from build123d import *

# Parameters (mm, degrees)
SKETCH1_W           = 700
SKETCH1_H           = 20
BOSS_EXTRUDE1_DEPTH = 2
FILLET1_R           = 9
SKETCH2_R           = 5
SKETCH2_R_2         = 2.25
CUT_EXTRUDE1_DEPTH  = 701.288511972


with BuildPart() as part:
    # Sketch1 → Boss-Extrude1 (new body)
    with BuildSketch(Plane(origin=(0, 0, 0), x_dir=(1, 0, 0), z_dir=(0, 1, 0))):
        with Locations((350, 10)):
            Rectangle(SKETCH1_W, SKETCH1_H)
    extrude(amount=BOSS_EXTRUDE1_DEPTH)

    # Fillet1
    fillet1_edges = [part.edges().sort_by_distance(p)[0] for p in [
        (0, 1, -20),
        (700, 1, -20),
        (700, 1, 0),
        (0, 1, 0),
    ]]
    fillet(fillet1_edges, radius=FILLET1_R)

    # Sketch2 → Cut-Extrude1 (cut, through all)
    with BuildSketch(Plane(origin=(0, 2, 0), x_dir=(1, 0, 0), z_dir=(0, 1, 0))):
        with Locations(Location((350, 10, 0), (0, 0, 270))):
            Circle(SKETCH2_R)
        with Locations(Location((130, 15, 0), (0, 0, 270))):
            Circle(SKETCH2_R_2)
        with Locations(Location((230, 15, 0), (0, 0, 270))):
            Circle(SKETCH2_R_2)
        with Locations(Location((130, 5, 0), (0, 0, 270))):
            Circle(SKETCH2_R_2)
        with Locations(Location((230, 5, 0), (0, 0, 270))):
            Circle(SKETCH2_R_2)
        with Locations(Location((470, 15, 0), (0, 0, 90))):
            Circle(SKETCH2_R_2)
        with Locations(Location((470, 5, 0), (0, 0, 90))):
            Circle(SKETCH2_R_2)
        with Locations(Location((570, 5, 0), (0, 0, 90))):
            Circle(SKETCH2_R_2)
        with Locations(Location((570, 15, 0), (0, 0, 90))):
            Circle(SKETCH2_R_2)
    extrude(amount=-CUT_EXTRUDE1_DEPTH, mode=Mode.SUBTRACT)


solid = part.part
Model file for the job. Use its own axes, mm. Coordinates: 2 decimals unless noted, no trailing zeros. Return JSON: item names as keys, results as strings. Group by question number.
Item 1: Wall check: line 1 along Z through (x, y) = (570, 1.4); line 2 along X through (y, z) = (1.55, -4); line 3 along X through (y, z) = (0.65, -16.5). Give the ranges that are in metal, low to high. Write a range as [from, to].
Item 2: Saw through at A-A on y = 0.7. State how many separate pieces and enclosed holes the cut face has, then the cut area to 3 significant figures.
Item 3: Flat gauge pins, fed straight in: P1, Ø4, axis at x = 230, z = -15, coming from the -Y side; P2, Ø5, axis at x = 470, z = -5, coming from the +Y side. Where does each tip first touch, or does it go through?
Values found:
{
 "1": {"line 1": "z = [-20, -17.25], [-12.75, -7.25], [-2.75, 0]", "line 2": "x = [1.52, 127.98], [132.02, 227.98], [232.02, 467.98], [472.02, 567.98], [572.02, 698.48]", "line 3": "x = [1.88, 128.32], [131.68, 228.32], [231.68, 468.32], [471.68, 568.32], [571.68, 698.12]"},
 "2": {"separate pieces": "1", "enclosed holes": "9", "area": "13,700 mm2"},
 "3": {"P1": "passes through", "P2": "stops at y = 2"}
}
